```python
from build123d import *

# Parameters (mm, degrees)
SKETCH1_W           = 27
SKETCH1_H           = 58
BOSS_EXTRUDE1_DEPTH = 2
BOSS_EXTRUDE2_DEPTH = 58
CUT_EXTRUDE1_DEPTH  = 58
SKETCH4_R           = 4
CUT_EXTRUDE2_DEPTH  = 58
CUT_EXTRUDE3_DEPTH  = 58
CUT_EXTRUDE4_DEPTH  = 58
SKETCH7_R           = 5
CUT_EXTRUDE5_DEPTH  = 58


with BuildPart() as part:
    # Sketch1 → Boss-Extrude1 (new body)
    with BuildSketch(Plane(origin=(0, 0, 0), x_dir=(1, 0, 0), z_dir=(0, 1, 0))):
        Rectangle(SKETCH1_W, SKETCH1_H)
    extrude(amount=BOSS_EXTRUDE1_DEPTH)

    # Sketch2 → Boss-Extrude2 (add)
    with BuildSketch(Plane.XY.offset(29)):
        with BuildLine():
            Line((-13.5, 2), (-13.5, 50))
            Line((-13.5, 50), (-11.5, 50))
            Line((-11.5, 50), (-11.5, 4))
            ThreePointArc((-11.5, 4), (-10.914213562, 2.585786438), (-9.5, 2))
            Line((-9.5, 2), (9.5, 2))
            ThreePointArc((9.5, 2), (10.914213562, 2.585786438), (11.5, 4))
            Line((11.5, 4), (11.5, 50))
            Line((11.5, 50), (13.5, 50))
            Line((13.5, 50), (13.5, 2))
            ThreePointArc((13.5, 2), (12.914213562, 0.585786438), (11.5, 0))
            Line((11.5, 0), (-11.5, 0))
            ThreePointArc((-11.5, 0), (-12.914213562, 0.585786438), (-13.5, 2))
        make_face()
    extrude(amount=-BOSS_EXTRUDE2_DEPTH)

    # Sketch3 → Cut-Extrude1 (cut)
    with BuildSketch(Plane(origin=(13.5, 0, 0), x_dir=(0, 0, -1), z_dir=(1, 0, 0))):
        Polygon((29, 17.261652863), (-29, 50), (29, 50), align=None)
    extrude(amount=-CUT_EXTRUDE1_DEPTH, mode=Mode.SUBTRACT)

    # Sketch4 → Cut-Extrude2 (cut)
    with BuildSketch(Plane(origin=(13.5, 0, 0), x_dir=(0, 0, -1), z_dir=(1, 0, 0))):
        with Locations((-21, 38)):
            Circle(SKETCH4_R)
    extrude(amount=-CUT_EXTRUDE2_DEPTH, mode=Mode.SUBTRACT)

    # Sketch5 → Cut-Extrude3 (cut)
    with BuildSketch(Plane(origin=(13.5, 0, 0), x_dir=(0, 0, -1), z_dir=(1, 0, 0))):
        with BuildLine():
            Line((-29, 41.436194465), (-29, 50))
            Line((-29, 50), (-21.542232449, 45.790431328))
            ThreePointArc((-21.542232449, 45.790431328), (-26.521027791, 45.754112815), (-29, 41.436194465))
        make_face()
    extrude(amount=-CUT_EXTRUDE3_DEPTH, mode=Mode.SUBTRACT)

    # Sketch6 → Cut-Extrude4 (cut)
    with BuildSketch(Plane.XY.offset(29)):
        with BuildLine():
            Line((-13.5, 0), (-11.5, 0))
            ThreePointArc((-11.5, 0), (-12.914213562, 0.585786438), (-13.5, 2))
            Line((-13.5, 2), (-13.5, 0))
        make_face()
        with BuildLine():
            Line((13.5, 2), (13.5, 0))
            Line((13.5, 0), (11.5, 0))
            ThreePointArc((11.5, 0), (12.914213562, 0.585786438), (13.5, 2))
        make_face()
    extrude(amount=-CUT_EXTRUDE4_DEPTH, mode=Mode.SUBTRACT)

    # Sketch7 → Cut-Extrude5 (cut)
    with BuildSketch(Plane.XZ):
        with Locations(Location((0, -11, 0), (0, 0, 270))):
            Circle(SKETCH7_R)
        with BuildLine():
            Line((-5, 19), (-5, 29))
            Line((-5, 29), (5, 29))
            Line((5, 29), (5, 19))
            ThreePointArc((5, 19), (0, 14), (-5, 19))
        make_face()
    extrude(amount=-CUT_EXTRUDE5_DEPTH, mode=Mode.SUBTRACT)


solid = part.part
```
Geometry check sheet. Reference: the model listing, model coordinates, mm. A direction names the side the tool comes from. Round coordinates to 2 decimals unless told otherwise and drop trailing zeros. Loops run counter-clockwise (first coordinate to the right, second up) from the corner with the lowest first, then second, coordinate; pieces in that order, holes last. Notation, with made-up numbers: (72, -10.5) - (91, -10.5) arc R30 cw to (91, 20.5) - close; hole circle Ø3 at (26, 61). An arc over 180 degrees is marked (long way). Write item = value, one per line. Start each with the question number.
1. Mould release check, pull along Z, two halves, no side actions. Record for faces 1 (the face through (1.5, 0.99, -15.77)), 2 (the face through (5, 1, 24)), 3 (the face through (-12.49, 31.33, -4.08)), 4 (the face through (-12, 18, 29)): released by +Z, released by -Z, zero draft, split by the parting line, or undercut.
2. Depth check by flat-ended pin: pin 1 (0.6 mm diameter, centred on y = 1, z = 24, fed in from -X); pin 2 (9.5 mm diameter, centred on x = -2.5, z = -5.5, fed in from +Y); pin 3 (0.6 mm diameter, centred on y = 1.5, z = 26, fed in from +X). Enter the tip coordinate at first touch or a pass-through.
3. Set-up check for faces 5 (the face through (-5, 1, 24)), 6 (the face through (12.51, 31.33, -4.08)), 7 (the face through (10.9, 2.57, 0.41)): record each of +Z, -Z, +X, -X, +Y, -Y from which the full face is reachable in a straight line by a thin tool's end or side.
4. Section check D-D on z = -11. Enter the section's corners in (x, y).
5. Thickness scan on line 1 (X direction, y = 18, z = 7); line 2 (Y direction, x = -6, z = -3.5); line 3 (Y direction, x = 12.35, z = 21). Record the ranges inside material, lowest first.
6. Section check B-B on y = 21.5. Enter the section's corners in (x, z).
7. Section check C-C on y = 38. Enter the section's corners in (x, z).
8. Section check A-A on x = 0. Enter the section's corners in (y, z).
Working result:
q1.face_1 = undercut
q1.face_2 = zero draft
q1.face_3 = released by -Z
q1.face_4 = released by +Z
q2.pin_1 = -13.37
q2.pin_2 = 2
q2.pin_3 = 13.49
q3.face_5 = +Z, +Y, -Y
q3.face_6 = -Z, +X, -X, +Y
q3.face_7 = +Z, -Z, +Y
q4.outline = (-13.5, 2) arc R2 ccw to (-11.5, 0) - (-5, 0) - (-5, 2) - (-9.5, 2) arc R2 cw to (-11.5, 4) - (-11.5, 27.42) - (-13.5, 27.42) - close; (5, 0) - (11.5, 0) arc R2 ccw to (13.5, 2) - (13.5, 27.42) - (11.5, 27.42) - (11.5, 4) arc R2 cw to (9.5, 2) - (5, 2) - close
q5.line_1 = -13.5 to -11.5, 11.5 to 13.5
q5.line_2 = 0 to 2
q5.line_3 = 0.19 to 34, 42 to 45.48
q6.outline = (-13.5, -21.49) - (-11.5, -21.49) - (-11.5, 29) - (-13.5, 29) - close; (11.5, -21.49) - (13.5, -21.49) - (13.5, 29) - (11.5, 29) - close
q7.outline = (-13.5, 7.74) - (-11.5, 7.74) - (-11.5, 17) - (-13.5, 17) - close; (-13.5, 25) - (-11.5, 25) - (-11.5, 29) - (-13.5, 29) - close; (11.5, 7.74) - (13.5, 7.74) - (13.5, 17) - (11.5, 17) - close; (11.5, 25) - (13.5, 25) - (13.5, 29) - (11.5, 29) - close
q8.outline = (0, -29) - (2, -29) - (2, -16) - (0, -16) - close; (0, -6) - (2, -6) - (2, 14) - (0, 14) - close
